```python
from build123d import *

# Parameters (mm, degrees)
BOSS_EXTRUDE1_DEPTH = 10
FILLET1_R           = 4
CHAMFER1_SIZE       = 1


with BuildPart() as part:
    # Sketch1 → Boss-Extrude1 (new body)
    with BuildSketch(Plane.XY):
        with BuildLine():
            Line((-12, 7.5), (28, 7.5))
            ThreePointArc((28, 7.5), (35.5, 0), (28, -7.5))
            Line((28, -7.5), (-12, -7.5))
            ThreePointArc((-12, -7.5), (-19.5, 0), (-12, 7.5))
        make_face()
        with BuildLine():
            Line((-0.5, -2), (0.5, -2))
            Line((0.5, -2), (0.5, -1.467140075))
            ThreePointArc((0.5, -1.467140075), (1.096015511, -1.096015511), (1.467140075, -0.5))
            Line((1.467140075, -0.5), (2, -0.5))
            Line((2, -0.5), (2, 0.5))
            Line((2, 0.5), (1.467140075, 0.5))
            ThreePointArc((1.467140075, 0.5), (1.096015511, 1.096015511), (0.5, 1.467140075))
            Line((0.5, 1.467140075), (0.5, 2))
            Line((0.5, 2), (-0.5, 2))
            Line((-0.5, 2), (-0.5, 1.467140075))
            ThreePointArc((-0.5, 1.467140075), (-1.096015511, 1.096015511), (-1.467140075, 0.5))
            Line((-1.467140075, 0.5), (-2, 0.5))
            Line((-2, 0.5), (-2, -0.5))
            Line((-2, -0.5), (-1.467140075, -0.5))
            ThreePointArc((-1.467140075, -0.5), (-1.096015511, -1.096015511), (-0.5, -1.467140075))
            Line((-0.5, -1.467140075), (-0.5, -2))
        make_face(mode=Mode.SUBTRACT)
        with BuildLine():
            Line((18, -0.5), (18, 0.5))
            Line((18, 0.5), (17.467140075, 0.5))
            ThreePointArc((17.467140075, 0.5), (17.096015511, 1.096015511), (16.5, 1.467140075))
            Line((16.5, 1.467140075), (16.5, 2))
            Line((16.5, 2), (15.5, 2))
            Line((15.5, 2), (15.5, 1.467140075))
            ThreePointArc((15.5, 1.467140075), (14.903984489, 1.096015511), (14.532859925, 0.5))
            Line((14.532859925, 0.5), (14, 0.5))
            Line((14, 0.5), (14, -0.5))
            Line((14, -0.5), (14.532859925, -0.5))
            ThreePointArc((14.532859925, -0.5), (14.903984489, -1.096015511), (15.5, -1.467140075))
            Line((15.5, -1.467140075), (15.5, -2))
            Line((15.5, -2), (16.5, -2))
            Line((16.5, -2), (16.5, -1.467140075))
            ThreePointArc((16.5, -1.467140075), (17.096015511, -1.096015511), (17.467140075, -0.5))
            Line((17.467140075, -0.5), (18, -0.5))
        make_face(mode=Mode.SUBTRACT)
    extrude(amount=BOSS_EXTRUDE1_DEPTH)

    # Fillet1
    fillet1_edges = [part.edges().sort_by_distance(p)[0] for p in [
        (35.5, 0, 10),
        (8, 7.5, 10),
        (-19.5, 0, 10),
        (8, -7.5, 10),
    ]]
    fillet(fillet1_edges, radius=FILLET1_R)

    # Chamfer1
    chamfer1_edges = [part.edges().sort_by_distance(p)[0] for p in [
        (8, 7.5, 0),
        (35.5, 0, 0),
        (8, -7.5, 0),
        (-19.5, 0, 0),
    ]]
    chamfer(chamfer1_edges, length=CHAMFER1_SIZE)


solid = part.part
```
Input: part model. Units: mm. Frame: model coordinates. A direction names the side the tool comes from. Round coordinates to 2 decimals unless told otherwise and drop trailing zeros. Write each loop counter-clockwise with the first axis right and the second up, starting at its lowest first coordinate (ties: lowest second). Pieces come first, ordered by that corner, then holes. Notation, with made-up numbers: M 60,-16.75 L 80,-16.75 A22 ccw 80,-3.75 Z; hole C -14.5,39.25 d10. An arc over 180 degrees is marked long. Write each question's results on one line, items separated by ' | '.
Q1. Line query: line 1 along X through (y, z) = (0, 4.5); line 2 along X through (y, z) = (1, 2.5); line 3 along Y through (x, z) = (-10.5, 6.25). Output: solid intervals per line, ascending.
Results:
line 1: x = -19.5 to -2, 2 to 14, 18 to 35.5 | line 2: x = -19.43 to -1.18, 1.18 to 14.82, 17.18 to 35.43 | line 3: y = -7.49 to 7.49
Q2. Section query A-A (x = -11). Return loops of the section in (y, z), and give its area (3 significant figures).
Results:
outline: M -7.5,1 L -6.5,0 L 6.5,0 L 7.5,1 L 7.5,6 A4 ccw 3.5,10 L -3.5,10 A4 ccw -7.5,6 Z | area: 142 mm^2
Q3. Section query B-B (z = 5). State how many separate pieces and enclosed holes the cut face has, and give its area (3 significant figures).
Results:
separate pieces: 1 | enclosed holes: 2 | area: 758 mm^2
Q4. Access query for faces 4 (the face through (17.09, -1.1, 4.93)), 5 (the face through (8, -7.5, 3)). Directions: +Z, -Z, +X, -X, +Y, -Y. A direction counts if a zero-diameter tool reaches every point of the face in a straight line with its end or side. Return the directions, or none.
Results:
face 4: +Z, -Z | face 5: +Z, -Z, +X, -X, -Y
Q5. Pin query (flat end, axial travel): P1, Ø0.6, axis at y = 1.5, z = 3, coming from the +X side; P2, Ø0.6, axis at y = -2, z = 3, coming from the +X side; P3, Ø2, axis at y = 2, z = 6.5, coming from the -X side. Return the tip coordinate at first contact, or that it passes through.
Results:
P1: stops at x = 35.4 | P2: stops at x = 35.3 | P3: stops at x = -19.42
Q6. Draft query along X for faces 1 (the face through (7.72, -6.359, 8.797)), 2 (the face through (0, 2, 5)), 3 (the face through (35.5, 0.16, 3.46)). Return one class per face: released by +X, released by -X, zero draft, split by the parting line, or undercut.
Results:
face 1: zero draft | face 2: undercut | face 3: released by +X
